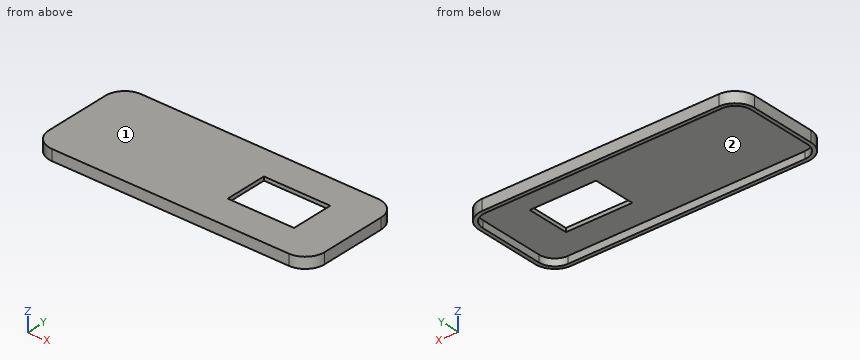
from build123d import *

# Parameters (mm, degrees)
SKETCH004_W      = 28
SKETCH004_H      = 18
EXTRUDE004_DEPTH = 1.6
EXTRUDE003_DEPTH = 3


with BuildPart() as obj1:
    # Sketch004 → Extrude004 (new body)
    with BuildSketch(Plane.XY):
        with BuildLine():
            Line((89.498192, -57.050084), (189.498192, -57.050084))
            ThreePointArc((197.698192, -65.250084), (195.296468, -59.451808), (189.498192, -57.050084))
            Line((197.698192, -65.250084), (197.698192, -93.250084))
            ThreePointArc((189.498192, -101.450084), (195.296468, -99.04836), (197.698192, -93.250084))
            Line((189.498192, -101.450084), (89.498192, -101.450084))
            ThreePointArc((81.298192, -93.250084), (83.699916, -99.04836), (89.498192, -101.450084))
            Line((81.298192, -93.250084), (81.298192, -65.250084))
            ThreePointArc((89.498192, -57.050084), (83.699916, -59.451808), (81.298192, -65.250084))
        make_face()
        with Locations((166.513474, -79.24515)):
            Rectangle(SKETCH004_W, SKETCH004_H, mode=Mode.SUBTRACT)
    extrude(amount=EXTRUDE004_DEPTH)


with BuildPart() as obj1_1:
    # Extrude004 placement: moved
    add(obj1.part.moved(Location((0, 0, 53))))


with BuildPart() as obj2:
    # Sketch003 → Extrude003 (new body)
    with BuildSketch(Plane.XY):
        with BuildLine():
            Line((89.498192, -57.050084), (189.498192, -57.050084))
            ThreePointArc((197.698192, -65.250084), (195.296468, -59.451808), (189.498192, -57.050084))
            Line((197.698192, -65.250084), (197.698192, -93.250084))
            ThreePointArc((189.498192, -101.450084), (195.296468, -99.04836), (197.698192, -93.250084))
            Line((189.498192, -101.450084), (89.498192, -101.450084))
            ThreePointArc((81.298192, -93.250084), (83.699916, -99.04836), (89.498192, -101.450084))
            Line((81.298192, -93.250084), (81.298192, -65.250084))
            ThreePointArc((89.498192, -57.050084), (83.699916, -59.451808), (81.298192, -65.250084))
        make_face()
        with BuildLine():
            Line((89.498192, -99.850084), (189.498192, -99.850084))
            ThreePointArc((189.498192, -99.850084), (194.165097, -97.916989), (196.098192, -93.250084))
            Line((196.098192, -93.250084), (196.098192, -65.250084))
            ThreePointArc((196.098192, -65.250084), (194.165097, -60.583179), (189.498192, -58.650084))
            Line((189.498192, -58.650084), (89.498192, -58.650084))
            ThreePointArc((89.498192, -58.650084), (84.831287, -60.583179), (82.898192, -65.250084))
            Line((82.898192, -65.250084), (82.898192, -93.250084))
            ThreePointArc((82.898192, -93.250084), (84.831287, -97.916989), (89.498192, -99.850084))
        make_face(mode=Mode.SUBTRACT)
    extrude(amount=EXTRUDE003_DEPTH)


with BuildPart() as obj2_1:
    # Extrude003 placement: moved
    add(obj2.part.moved(Location((0, 0, 50))))

    # Fusion001: union obj1
    add(obj1_1.part)


solid = obj2_1.part
For this review, take the finished solid that the model builds, in its own axes (mm). Face numbers are marked on the shaded views. Coordinates: 2 decimals unless noted, no trailing zeros. Loops run counter-clockwise (first coordinate to the right, second up) from the corner with the lowest first, then second, coordinate; pieces in that order, holes last. Notation, with made-up numbers: (33, -38) - (78, -38) arc R27 ccw to (78, -13) - close; hole circle Ø7 at (6, 39.5). An arc over 180 degrees is marked (long way). Return JSON: item names as keys, results as strings.
Item 1: Insertion check: pin 1 (5 mm diameter, centred on x = 128.5, y = -79.5, fed in from -Z); pin 2 (1 mm diameter, centred on y = -95, z = 53, fed in from -X). Each pin has a flat end and moves straight along its axis. Give the tip position at first contact, or say it passes through.
Determined:
{"pin 1": "stops at z = 53", "pin 2": "stops at x = 81.39"}
Item 2: Take a section at A-A (z = 53.85). Give the boundary of the cut face in (x, y).
Determined:
{"outline": "(81.3, -93.25) arc R8.2 ccw to (89.5, -101.45) - (189.5, -101.45) arc R8.2 ccw to (197.7, -93.25) - (197.7, -65.25) arc R8.2 ccw to (189.5, -57.05) - (89.5, -57.05) arc R8.2 ccw to (81.3, -65.25) - close; hole (152.51, -88.25) - (180.51, -88.25) - (180.51, -70.25) - (152.51, -70.25) - close"}
Item 3: Take a section at D-D (x = 125). Give the boundary of the cut face in (y, z), then the cut area to 3 significant figures.
Determined:
{"outline": "(-101.45, 50) - (-99.85, 50) - (-99.85, 53) - (-58.65, 53) - (-58.65, 50) - (-57.05, 50) - (-57.05, 54.6) - (-101.45, 54.6) - close", "area": "80.6 mm2"}
Item 4: For line 1 (X direction, y = -87.5, z = 53.65); line 2 (X direction, y = -72.5, z = 52.2); line 3 (Y direction, x = 113.5, z = 50.3), list the stretches that pass through material, from the lowest coordinate up.
Determined:
{"line 1": "x = 81.3 to 152.51, 180.51 to 197.7", "line 2": "x = 81.3 to 82.9, 196.1 to 197.7", "line 3": "y = -101.45 to -99.85, -58.65 to -57.05"}
Item 5: Take a section at B-B (y = -79.5). Give the boundary of the cut face in (x, z).
Determined:
{"outline": "(81.3, 50) - (82.9, 50) - (82.9, 53) - (152.51, 53) - (152.51, 54.6) - (81.3, 54.6) - close; (180.51, 53) - (196.1, 53) - (196.1, 50) - (197.7, 50) - (197.7, 54.6) - (180.51, 54.6) - close"}
Item 6: Mouldability with a two-part tool opening along Y and no side actions: class the marked faces 1 and 2 as pulls with the +Y half, pulls with the -Y half, needs draft (parallel to the pull), parting line crosses it, or undercut.
Determined:
{"face 1": "needs draft", "face 2": "undercut"}
Item 7: Take a section at C-C (x = 179). Give the boundary of the cut face in (y, z).
Determined:
{"outline": "(-101.45, 50) - (-99.85, 50) - (-99.85, 53) - (-88.25, 53) - (-88.25, 54.6) - (-101.45, 54.6) - close; (-70.25, 53) - (-58.65, 53) - (-58.65, 50) - (-57.05, 50) - (-57.05, 54.6) - (-70.25, 54.6) - close"}
